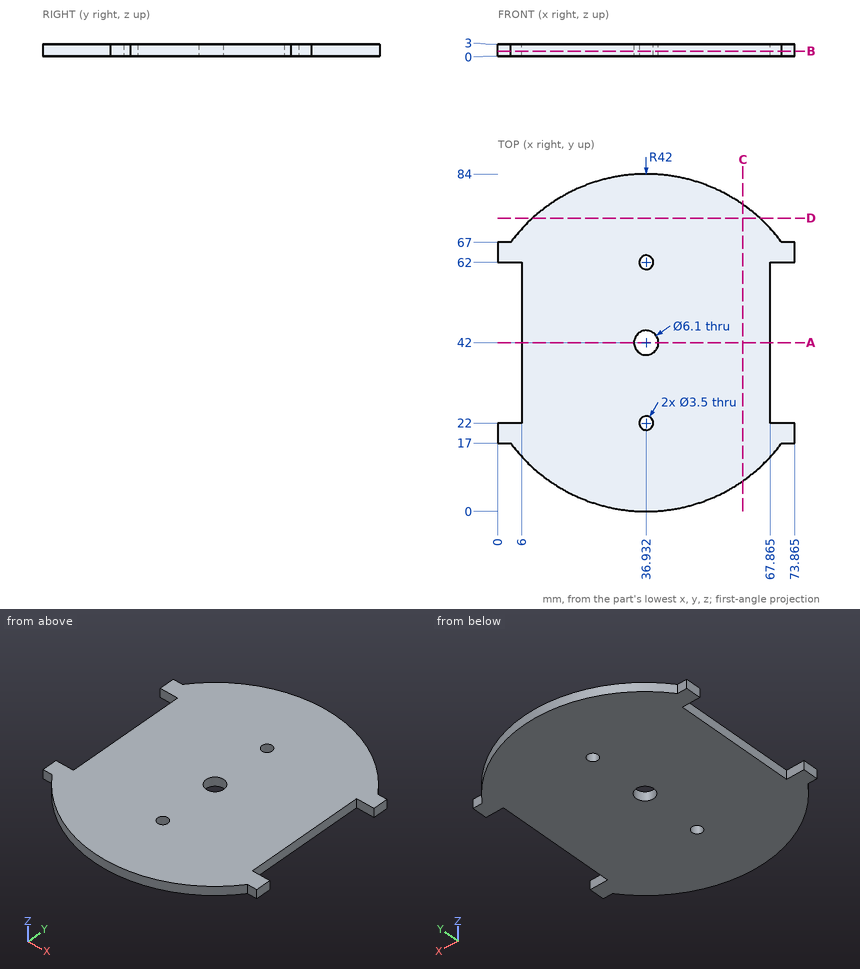
Job drawing, mm, ordinate dimensions from the low corner. One solid piece. Coordinates: 2 decimals unless noted, no trailing zeros. Write each loop counter-clockwise with the first axis right and the second up, starting at its lowest first coordinate (ties: lowest second). Pieces come first, ordered by that corner, then holes. Notation, with made-up numbers: M 8.5,-39.5 L 37.5,-39.5 A17 cw 37.5,-19.5 Z; hole C -19.75,27.5 d8. An arc over 180 degrees is marked long. Answer as a JSON object with one key per item and string values. Group by question number.
1) Wall check: line 1 (X direction, y = 57.5, z = 0.95) (1 decimal); line 2 (Y direction, x = 71.5, z = 1.25); line 3 (Y direction, x = 70, z = 2.45) (1 decimal). Give the ranges that are in metal, low to high. Write a range as from..to.
2) Saw through at D-D (y = 73). Write the cut outline in (x, z) (1 decimal).
3) Saw through at C-C (x = 61). Write the cut outline in (y, z).
4) Saw through at A-A (y = 42). Write the cut outline in (x, z) (1 decimal).
5) Saw through at B-B (z = 1.2). Give the number of separate pieces and of enclosed holes in the cut face, plus the area to 3 significant figures.
6) Pin check, flat tips, straight feed: pin 1 Ø1.5 at (y, z) = (24.5, 0.5) entering from +X (1 decimal); pin 2 Ø0.9 at (x, z) = (3.5, 2) entering from +Y; pin 3 Ø1 at (y, z) = (50.5, 1.5) entering from -X. Stop position of each tip, or through.
Values follow:
{
 "1": {"line 1": "x = 6..67.9", "line 2": "y = 17..22, 62..67", "line 3": "y = 16.1..22, 62..67.9"},
 "2": {"outline": "M 8.6,0 L 65.3,0 L 65.3,3 L 8.6,3 Z"},
 "3": {"outline": "M 7.58,0 L 76.42,0 L 76.42,3 L 7.58,3 Z"},
 "4": {"outline": "M 6,0 L 33.9,0 L 33.9,3 L 6,3 Z; M 40,0 L 67.9,0 L 67.9,3 L 40,3 Z"},
 "5": {"separate pieces": "1", "enclosed holes": "3", "area": "4,770 mm2"},
 "6": {"pin 1": "stops at x = 67.9", "pin 2": "stops at y = 68", "pin 3": "stops at x = 6"}
}
